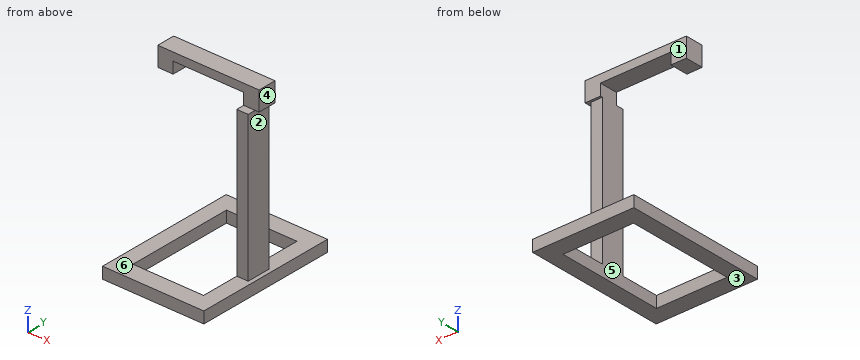
```python
from build123d import *

# Parameters (mm, degrees)
SKETCH1_W           = 89.004906374
SKETCH1_H           = 124.399859706
SKETCH1_W_2         = 61.999445932
SKETCH1_H_2         = 93.995967372
BOSS_EXTRUDE1_DEPTH = 10
SKETCH2_W           = 9.996534877
SKETCH2_H           = 20.999060591
BOSS_EXTRUDE2_DEPTH = 128
SKETCH3_W           = 89.004906374
SKETCH3_H           = 124.399859706
SKETCH3_W_2         = 61.999445932
SKETCH3_H_2         = 93.995967372
BOSS_EXTRUDE3_DEPTH = 17
SKETCH4_W           = 61.999445932
SKETCH4_H           = 16.009834455
BOSS_EXTRUDE4_DEPTH = 7
SKETCH5_W           = 89.004906374
SKETCH5_H           = 55.583620716
SKETCH5_H_2         = 52.806404535
CUT_EXTRUDE1_DEPTH  = 17


with BuildPart() as part:
    # Sketch1 → Boss-Extrude1 (new body)
    with BuildSketch(Plane.XY):
        Rectangle(SKETCH1_W, SKETCH1_H)
        Rectangle(SKETCH1_W_2, SKETCH1_H_2, mode=Mode.SUBTRACT)
    extrude(amount=BOSS_EXTRUDE1_DEPTH)

    # Sketch2 → Boss-Extrude2 (add)
    with BuildSketch(Plane.XY.offset(10)):
        with Locations((35.997990405, -3.066392871)):
            Rectangle(SKETCH2_W, SKETCH2_H)
    extrude(amount=BOSS_EXTRUDE2_DEPTH)

    # Sketch3 → Boss-Extrude3 (add)
    with BuildSketch(Plane.XY.offset(138)):
        Rectangle(SKETCH3_W, SKETCH3_H)
        Rectangle(SKETCH3_W_2, SKETCH3_H_2, mode=Mode.SUBTRACT)
    extrude(amount=BOSS_EXTRUDE3_DEPTH)

    # Sketch4 → Boss-Extrude4 (add)
    with BuildSketch(Plane.XY.offset(155)):
        with Locations((0, 1.388608091)):
            Rectangle(SKETCH4_W, SKETCH4_H)
    extrude(amount=-BOSS_EXTRUDE4_DEPTH)

    # Sketch5 → Cut-Extrude1 (cut)
    with BuildSketch(Plane.XY.offset(155)):
        with Locations((0, -34.408119495)):
            Rectangle(SKETCH5_W, SKETCH5_H)
        with Locations((0, 35.796727586)):
            Rectangle(SKETCH5_W, SKETCH5_H_2)
    extrude(amount=-CUT_EXTRUDE1_DEPTH, mode=Mode.SUBTRACT)


solid = part.part
```
The model under review builds one solid part; all positions refer to its coordinate system, in mm. Face numbers are marked on the shaded views. A direction names the side the tool comes from. Give positions to 0.01 mm unless a question says otherwise; leave off trailing zeros. Order: outer loops, then holes, each group sorted by start corner. A loop starts at its lowest first (then second) coordinate and runs counter-clockwise, first axis right, second up. Notation, with made-up numbers: (13, 31) - (56, 31) arc R17 ccw to (56, 37) - close; hole circle Ø5 at (6.5, 0). An arc over 180 degrees is marked (long way). Use CSV: the item, a comma, the result in double quotes. Start each with the question number.
Q1. We need section C-C, the plane x = 37.5. Write out the cut boundary in (y, z).
Q2. Clearance check with flat-ended pins moving along their axes: pin 1 Ø5 at (x, y) = (4, 2) entering from -Z; pin 2 Ø23 at (y, z) = (-1, 53.5) entering from +X; pin 3 Ø13.5 at (x, z) = (-12.5, 146.5) entering from +Y. State where each tip first meets the part, or that it passes through.
Q3. We need section A-A, the plane x = -3. Write out the cut boundary in (y, z), and give its area (3 significant figures).
Q4. The part is to be moulded in two halves that separate along X. For the marked faces 4, 5 and 6, say which applies: +X half, -X half, draft (parallel to the pull), parting line (faces both ways), or undercut.
Q5. We need section D-D, the plane x = -35. Write out the cut boundary in (y, z).
Q6. We need section B-B, the plane y = -21.5. Write out the cut boundary in (x, z), and give its area (3 significant figures).
Q7. To check wall thickness, follow line 1 along X through (y, z) = (-1.5, 139); line 2 along Z through (x, y) = (-32.5, 21.5); line 3 along Z through (x, y) = (-13.5, 5.5). State the ranges of each line that lie inside material, in increasing order. Write a range as [from, to].
Q8. Tool access review of the marked faces 1, 2 and 3: name each direction out of +Z, -Z, +X, -X, +Y, -Y from which nothing blocks a thin tool from reaching the whole face with its end or side.
Outcome:
1,outline,"(-62.2, 0) - (62.2, 0) - (62.2, 10) - (7.43, 10) - (7.43, 138) - (9.39, 138) - (9.39, 155) - (-6.62, 155) - (-6.62, 138) - (-13.57, 138) - (-13.57, 10) - (-62.2, 10) - close"
2,pin 1,"stops at z = 148"
2,pin 2,"stops at x = 41"
2,pin 3,"stops at y = 9.39"
3,outline,"(-62.2, 0) - (-47, 0) - (-47, 10) - (-62.2, 10) - close; (-6.62, 148) - (9.39, 148) - (9.39, 155) - (-6.62, 155) - close; (47, 0) - (62.2, 0) - (62.2, 10) - (47, 10) - close"
3,area,"416 mm^2"
4,face 4,"+X half"
4,face 5,"undercut"
4,face 6,"draft"
5,outline,"(-62.2, 0) - (62.2, 0) - (62.2, 10) - (-62.2, 10) - close; (-6.62, 138) - (9.39, 138) - (9.39, 155) - (-6.62, 155) - close"
6,outline,"(-44.5, 0) - (-31, 0) - (-31, 10) - (-44.5, 10) - close; (31, 0) - (44.5, 0) - (44.5, 10) - (31, 10) - close"
6,area,"270 mm^2"
7,line 1,"x = [-44.5, -31], [31, 44.5]"
7,line 2,"z = [0, 10]"
7,line 3,"z = [148, 155]"
8,face 1,"+Z, +X, -X, +Y"
8,face 2,"+X, +Y, -Y"
8,face 3,"-Z, +X, -X, +Y, -Y"
